```python
from build123d import *

# Parameters (mm, degrees)
SKETCH_1_W          = 16
SKETCH_1_H          = 6
EXTRUDE_1_DEPTH     = 0.4
SKETCH_2_W          = 16
SKETCH_2_H          = 6
EXTRUDE_2_DEPTH     = 3
EXTRUDE_2_TAPER     = 6
SKETCH_3_W          = 16
SKETCH_3_H          = 6
EXTRUDE_3_DEPTH     = 1.5
EXTRUDE_3_TAPER     = 3
CUT_EXTRUDE_4_DEPTH = 0.5
EXTRUDE_1_2_DEPTH   = 1.2
CUT_EXTRUDE_START   = -0.254
CUT_EXTRUDE_5_DEPTH = 0.254


# Read off the part's stored shape, not the designer's step: 伸長-薄件1
with BuildPart() as part:
    # 草圖1 → Extrude 1 (new body)
    with BuildSketch(Plane(origin=(0, 0, 0), x_dir=(1, 0, 0), z_dir=(0, 1, 0))):
        with Locations((7, 0)):
            Rectangle(SKETCH_1_W, SKETCH_1_H)
    extrude(amount=EXTRUDE_1_DEPTH)

    # 草圖2 → 伸長2 (add)
    with BuildSketch(Plane(origin=(0, 0.4, 0), x_dir=(1, 0, 0), z_dir=(0, 1, 0))):
        with Locations((7, 0)):
            Rectangle(SKETCH_2_W, SKETCH_2_H)
    extrude(amount=EXTRUDE_2_DEPTH, taper=EXTRUDE_2_TAPER)

    # 草圖3 → 伸長3 (add)
    with BuildSketch(Plane(origin=(0, 0, 0), x_dir=(-1, 0, 0), z_dir=(0, -1, 0))):
        with Locations((-7, 0)):
            Rectangle(SKETCH_3_W, SKETCH_3_H)
    extrude(amount=EXTRUDE_3_DEPTH, taper=EXTRUDE_3_TAPER)

    # 草圖4 → 伸長4 (cut)
    with BuildSketch(Plane(origin=(0, 3.4, 0), x_dir=(1, 0, 0), z_dir=(0, 1, 0))):
        with BuildLine():
            Line((-1, 0.8), (1.5, 0.8))
            ThreePointArc((1.5, 0.8), (2.3, 0), (1.5, -0.8))
            Line((1.5, -0.8), (-1, -0.8))
            Line((-1, -0.8), (-1, 0.8))
        make_face()
    extrude(amount=-CUT_EXTRUDE_4_DEPTH, mode=Mode.SUBTRACT)

    # Extrude 1 2 outline → Extrude 1 2 (add)
    with BuildSketch(Plane(origin=(0, 0, 0), x_dir=(0, 0, -1), z_dir=(1, 0, 0))):
        with BuildLine():
            Line((-3, 0.2), (-3, 0.454))
            Line((-3, 0.454), (-3.8, 0.454))
            ThreePointArc((-3.8, 0.454), (-4.121026479, 0.321026479), (-4.254, 0))
            Line((-4.254, 0), (-4.254, -4.8))
            Line((-4.254, -4.8), (-4, -4.8))
            Line((-4, -4.8), (-4, 0))
            ThreePointArc((-4, 0), (-3.941421356, 0.141421356), (-3.8, 0.2))
            Line((-3.8, 0.2), (-3, 0.2))
        make_face()
    extrude(amount=EXTRUDE_1_2_DEPTH)

    # 草圖6 → 伸長5 (cut)
    with BuildSketch(Plane.XY.offset(4.254).offset(CUT_EXTRUDE_START)):
        Polygon((0.6, -4.8), (0.823031072, -4.518152134), (0.823031072, -1.899802565), (1.593384633, -1.289166003), (1.593384633, -5.180880526), (-0.393384633, -5.180880526), (-0.393384633, -1.289166003), (0.376968928, -1.899802565), (0.376968928, -4.518152134), align=None)
    extrude(amount=CUT_EXTRUDE_5_DEPTH, mode=Mode.SUBTRACT)


solid = part.part
```
The listing builds one solid part. Answer for the finished solid, in the listing's coordinates (mm). A direction names the side the tool comes from. Give positions to 0.01 mm unless a question says otherwise; leave off trailing zeros. Answer in a Markdown table with one row per item. Add a question column.
Q1. Find the intervals of material crossed by line 1 along Z through (x, y) = (3, 0); line 2 along Y through (x, z) = (0, 0.5); line 3 along Z through (x, y) = (0.75, 3.25), in increasing order. Write a range as [from, to].
Q2. Which of the six approach directions +Z, -Z, +X, -X, +Y, -Y give full straight-line access (tool end or side, diameter ignored) to faces 1 (the flat face through (0.6, -1.9, 4)), 2 (the flat face through (1, 2.9, 0)), 3 (the flat face through (0.6, -1.8, 4.254))?
Q3. Given P1, Ø0.6, axis at y = -0.5, z = 4, coming from the -X side; P2, Ø0.8, axis at x = 1.5, z = 0, coming from the +Y side; P3, Ø1, axis at y = 1.5, z = -2, coming from the +X side; P4, Ø1.5, axis at y = 0.5, z = 2.5, coming from the -X side, each flat-ended and moving along its own axis, determine where each tip first touches the part or whether it passes through.
Determined:
| question | item | result |
|---|---|---|
| 1 | line 1 | z = [-3, 3] |
| 1 | line 2 | y = [-1.5, 2.9] |
| 1 | line 3 | z = [-2.7, -0.8], [0.8, 2.7] |
| 2 | face 1 | +X, -X, -Y |
| 2 | face 2 | -X, +Y |
| 2 | face 3 | +Z, +X, -X, +Y, -Y |
| 3 | P1 | stops at x = 0 |
| 3 | P2 | stops at y = 2.9 |
| 3 | P3 | stops at x = 14.94 |
| 3 | P4 | stops at x = -1 |
